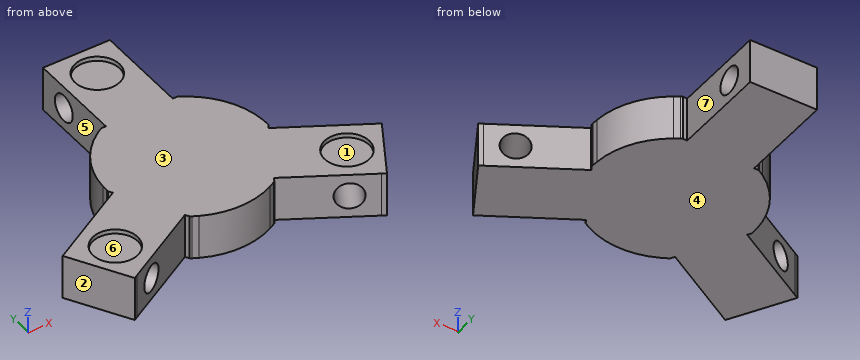
from build123d import *
from build123d.topology import SkipClean

# Parameters (mm, degrees)
EXTRUDE_1_DEPTH      = 5
SKETCH_2_R           = 1.5
CUT_EXTRUDE_1_DEPTH  = 10
SKETCH_3_R           = 1.5
CUT_EXTRUDE_2_DEPTH  = 10
SKETCH_4_R           = 1.5
CUT_EXTRUDE_3_DEPTH  = 10
CUT_EXTRUDE_4_DEPTH  = 3
SKETCH_6_R           = 2.5
CUT_EXTRUDE_5_DEPTH  = 5
CUT_EXTRUDE_START    = -10
CUT_EXTRUDE_6_DEPTH  = 10
SKETCH_9_R           = 2.9
CUT_EXTRUDE_7_DEPTH  = 10
CUT_EXTRUDE_8_DEPTH  = 10
SKETCH_12_R          = 2.5
CUT_EXTRUDE_10_DEPTH = 0.5
SKETCH_13_R          = 5.742346741
EXTRUDE_2_DEPTH      = 5
SKETCH_14_W          = 0.5
SKETCH_14_H          = 10.069998948
CUT_EXTRUDE_11_DEPTH = 5
SKETCH_16_W          = 7.5
SKETCH_16_H          = 0.5
EXTRUDE_3_DEPTH      = 5


with BuildPart() as part:
    # 草图1 → 凸台-拉伸1 (new body)
    with BuildSketch(Plane.XY):
        with BuildLine():
            Line((8.980740698, 0.588469632), (18.088457268, -4.669872981))
            Line((18.088457268, -4.669872981), (13.088457268, -13.330127019))
            Line((13.088457268, -13.330127019), (3.980740698, -8.071784406))
            ThreePointArc((3.980740698, -8.071784406), (0, -9), (-3.980740698, -8.071784406))
            Line((-3.980740698, -8.071784406), (-13.088457268, -13.330127019))
            Line((-13.088457268, -13.330127019), (-18.088457268, -4.669872981))
            Line((-18.088457268, -4.669872981), (-8.980740698, 0.588469632))
            ThreePointArc((-8.980740698, 0.588469632), (-7.794228634, 4.5), (-5, 7.483314774))
            Line((-5, 7.483314774), (-5, 18.003314774))
            Line((-5, 18.003314774), (5, 18.003314774))
            Line((5, 18.003314774), (5, 7.483314774))
            ThreePointArc((5, 7.483314774), (7.794228634, 4.5), (8.980740698, 0.588469632))
        make_face()
    extrude(amount=EXTRUDE_1_DEPTH)

    # 草图2 → 切除-拉伸1 (cut)
    with BuildSketch(Plane(origin=(5, 0, 0), x_dir=(0, 0, -1), z_dir=(1, 0, 0))):
        with Locations(Location((-2.5, 15.003314774, 0), (0, 0, 90))):
            Circle(SKETCH_2_R)
    extrude(amount=-CUT_EXTRUDE_1_DEPTH, mode=Mode.SUBTRACT)

    # 草图3 → 切除-拉伸2 (cut)
    with BuildSketch(Plane(origin=(-2.5, -4.330127019, 0), x_dir=(0.8660254037844364, -0.5000000000000041, 0), z_dir=(-0.500000000000004, -0.8660254037844363, 0))):
        with Locations((15, 2.5)):
            Circle(SKETCH_3_R)
    extrude(amount=-CUT_EXTRUDE_2_DEPTH, mode=Mode.SUBTRACT)

    # 草图4 → 切除-拉伸3 (cut)
    with BuildSketch(Plane(origin=(2.5, -4.330127019, 0), x_dir=(0.8660254037844434, 0.49999999999999184, 0), z_dir=(0.49999999999999184, -0.8660254037844434, 0))):
        with Locations((-15, 2.5)):
            Circle(SKETCH_4_R)
    extrude(amount=-CUT_EXTRUDE_3_DEPTH, mode=Mode.SUBTRACT)

    # 草图5 → 切除-拉伸4 (cut)
    with BuildSketch(Plane.XY.offset(5)):
        Polygon((-4, 0), (-2, -3.464101615), (2, -3.464101615), (4, 0), (2, 3.464101615), (-2, 3.464101615), align=None)
    extrude(amount=-CUT_EXTRUDE_4_DEPTH, mode=Mode.SUBTRACT)

    # 草图6 → 切除-拉伸5 (cut)
    with BuildSketch(Plane.XY.offset(5)):
        Circle(SKETCH_6_R)
    extrude(amount=-CUT_EXTRUDE_5_DEPTH, mode=Mode.SUBTRACT)

    # 草图8 → 切除-拉伸6 (cut)
    with SkipClean():  # the faces are left unmerged after this step: merging them gives an invalid solid
        with BuildSketch(Plane.XY.offset(5).offset(CUT_EXTRUDE_START)):
            with BuildLine():
                Line((-8.999815496, -0.057628503), (-17.813457268, -5.146186953))
                Line((-17.813457268, -5.146186953), (-18.088457268, -4.669872981))
                Line((-18.088457268, -4.669872981), (-8.980740698, 0.588469632))
                ThreePointArc((-8.980740698, 0.588469632), (-8.996080311, 0.265591864), (-8.999815496, -0.057628503))
            make_face()
            with BuildLine():
                Line((-4.549815496, -7.765254597), (-13.363457268, -12.853813047))
                Line((-13.363457268, -12.853813047), (-13.088457268, -13.330127019))
                Line((-13.088457268, -13.330127019), (-3.980740698, -8.071784406))
                ThreePointArc((-3.980740698, -8.071784406), (-4.268030855, -7.923630016), (-4.549815496, -7.765254597))
            make_face()
            with BuildLine():
                Line((-4.45, 7.8228831), (-4.45, 18.003314774))
                Line((-4.45, 18.003314774), (-5, 18.003314774))
                Line((-5, 18.003314774), (-5, 7.483314774))
                ThreePointArc((-5, 7.483314774), (-4.728049456, 7.658038152), (-4.45, 7.8228831))
            make_face()
            with BuildLine():
                Line((4.45, 7.8228831), (4.45, 18.003314774))
                Line((4.45, 18.003314774), (5, 18.003314774))
                Line((5, 18.003314774), (5, 7.483314774))
                ThreePointArc((5, 7.483314774), (4.728049456, 7.658038152), (4.45, 7.8228831))
            make_face()
            with BuildLine():
                Line((4.549815496, -7.765254597), (13.363457268, -12.853813047))
                Line((13.363457268, -12.853813047), (13.088457268, -13.330127019))
                Line((13.088457268, -13.330127019), (3.980740698, -8.071784406))
                ThreePointArc((3.980740698, -8.071784406), (4.268030855, -7.923630016), (4.549815496, -7.765254597))
            make_face()
            with BuildLine():
                Line((8.999815496, -0.057628503), (17.813457268, -5.146186953))
                Line((17.813457268, -5.146186953), (18.088457268, -4.669872981))
                Line((18.088457268, -4.669872981), (8.980740698, 0.588469632))
                ThreePointArc((8.980740698, 0.588469632), (8.996080311, 0.265591864), (8.999815496, -0.057628503))
            make_face()
        extrude(amount=CUT_EXTRUDE_6_DEPTH, mode=Mode.SUBTRACT)

    # 草图9 → 切除-拉伸7 (cut)
    with SkipClean():  # the faces are left unmerged after this step: merging them gives an invalid solid
        with BuildSketch(Plane(origin=(0, 0, 0), x_dir=(-1, 0, 0), z_dir=(0, 0, -1))):
            Circle(SKETCH_9_R)
        extrude(amount=-CUT_EXTRUDE_7_DEPTH, mode=Mode.SUBTRACT)

    # 草图11 → 切除-拉伸8 (cut)
    with BuildSketch(Plane.XY.offset(5).offset(CUT_EXTRUDE_START)):
        with BuildLine():
            Line((17.813457268, -5.146186953), (17.713457268, -5.319392034))
            Line((17.713457268, -5.319392034), (8.995453042, -0.286049947))
            ThreePointArc((8.995453042, -0.286049947), (8.998359102, -0.171853068), (8.999815496, -0.057628503))
            Line((8.999815496, -0.057628503), (17.813457268, -5.146186953))
        make_face()
        with BuildLine():
            Line((-4.45, 18.003314774), (-4.25, 18.003314774))
            Line((-4.25, 18.003314774), (-4.25, 7.933315826))
            ThreePointArc((-4.25, 7.933315826), (-4.350350428, 7.878734109), (-4.45, 7.8228831))
            Line((-4.45, 7.8228831), (-4.45, 18.003314774))
        make_face()
        with BuildLine():
            Line((4.45, 18.003314774), (4.45, 7.8228831))
            ThreePointArc((4.45, 7.8228831), (4.350350428, 7.878734109), (4.25, 7.933315826))
            Line((4.25, 7.933315826), (4.25, 18.003314774))
            Line((4.25, 18.003314774), (4.45, 18.003314774))
        make_face()
        with BuildLine():
            Line((13.363457268, -12.853813047), (4.549815496, -7.765254597))
            ThreePointArc((4.549815496, -7.765254597), (4.648008674, -7.70688104), (4.745453042, -7.647265879))
            Line((4.745453042, -7.647265879), (13.463457268, -12.680607966))
            Line((13.463457268, -12.680607966), (13.363457268, -12.853813047))
        make_face()
        with BuildLine():
            Line((-4.549815496, -7.765254597), (-13.363457268, -12.853813047))
            Line((-13.363457268, -12.853813047), (-13.463457268, -12.680607966))
            Line((-13.463457268, -12.680607966), (-4.745453042, -7.647265879))
            ThreePointArc((-4.745453042, -7.647265879), (-4.648008674, -7.70688104), (-4.549815496, -7.765254597))
        make_face()
        with BuildLine():
            Line((-17.813457268, -5.146186953), (-17.713457268, -5.319392034))
            Line((-17.713457268, -5.319392034), (-8.995453042, -0.286049947))
            ThreePointArc((-8.995453042, -0.286049947), (-8.998359102, -0.171853068), (-8.999815496, -0.057628503))
            Line((-8.999815496, -0.057628503), (-17.813457268, -5.146186953))
        make_face()
    extrude(amount=CUT_EXTRUDE_8_DEPTH, mode=Mode.SUBTRACT)

    # 草图12 → 切除-拉伸10 (cut)
    with BuildSketch(Plane.XY.offset(5)):
        with Locations((0, 15)):
            Circle(SKETCH_12_R)
        with Locations((12.990381057, -7.5)):
            Circle(SKETCH_12_R)
        with Locations((-12.990381057, -7.5)):
            Circle(SKETCH_12_R)
    extrude(amount=-CUT_EXTRUDE_10_DEPTH, mode=Mode.SUBTRACT)

    # 草图13 → 凸台-拉伸2 (add)
    with BuildSketch(Plane.XY.offset(5)):
        Circle(SKETCH_13_R)
    extrude(amount=-EXTRUDE_2_DEPTH)

    # 草图14 → 切除-拉伸11 (cut)
    with BuildSketch(Plane.XY.offset(5)):
        with Locations((-4, 12.9683153)):
            Rectangle(SKETCH_14_W, SKETCH_14_H)
        with Locations((4, 12.9683153)):
            Rectangle(SKETCH_14_W, SKETCH_14_H)
        Polygon((-17.463457268, -5.752404736), (-8.745453042, -0.719062649), (-8.995453042, -0.286049947), (-17.713457268, -5.319392034), align=None)
        Polygon((-4.995453042, -7.214253177), (-13.713457268, -12.247595264), (-13.463457268, -12.680607966), (-4.745453042, -7.647265879), align=None)
        Polygon((13.713457268, -12.247595264), (4.995453042, -7.214253177), (4.745453042, -7.647265879), (13.463457268, -12.680607966), align=None)
        Polygon((8.745453042, -0.719062649), (17.463457268, -5.752404736), (17.713457268, -5.319392034), (8.995453042, -0.286049947), align=None)
    extrude(amount=-CUT_EXTRUDE_11_DEPTH, mode=Mode.SUBTRACT)

    # 草图16 → 凸台-拉伸3 (add)
    with BuildSketch(Plane.XY.offset(5)):
        with Locations((0, 18.253314774)):
            Rectangle(SKETCH_16_W, SKETCH_16_H)
        Polygon((-17.89646997, -6.002404736), (-14.14646997, -12.497595264), (-13.713457268, -12.247595264), (-17.463457268, -5.752404736), align=None)
        Polygon((17.89646997, -6.002404736), (14.14646997, -12.497595264), (13.713457268, -12.247595264), (17.463457268, -5.752404736), align=None)
    extrude(amount=-EXTRUDE_3_DEPTH)


solid = part.part
Could you check a few things on this model? Use its own coordinates, in mm. Face numbers are marked on the shaded views. A direction names the side the tool comes from. Coordinates: 2 decimals unless noted, no trailing zeros. Order: outer loops, then holes, each group sorted by start corner. A loop starts at its lowest first (then second) coordinate and runs counter-clockwise, first axis right, second up. Notation, with made-up numbers: (41.5, -19.5) - (64.5, -19.5) arc R31 cw to (64.5, 18.5) - close; hole circle Ø9 at (69, -16). An arc over 180 degrees is marked (long way). Answer in a Markdown table with one row per item. Add a question column.
(1) If we section it at C-C, the plane z = 0.45: Please give me the cut outline in (x, y).
(2) If we section it at B-B, the plane y = 15: Please give me the cut outline in (x, z).
(3) On a 3-axis mill with a long thin cutter (end or side, diameter ignored), from which of +Z, -Z, +X, -X, +Y, -Y can I reach the whole of each face in a straight line? I mean the marked faces 4, 5, 6 and 7. Say none if no direction works.
(4) If we section it at A-A, the plane x = 0: Please give me the cut outline in (y, z).
(5) If we mould it in two halves opening along Y, with no side actions, what happens to the marked faces 1, 2 and 3? For each: released by +Y, released by -Y, zero draft, split by the parting line, or undercut.
(6) I need wall thicknesses on L1, parallel to X at y = 16.5, z = 3.05; L2, parallel to Y at x = -2, z = 1.35; L3, parallel to X at y = 5.5, z = 0.65. Which ranges of each line are inside material? Lowest first, please.
(7) If we section it at D-D, the plane z = 2.5: State how many separate pieces and enclosed holes the cut face has, then the cut area to 3 significant figures.
(8) Will these pins go through, and if not, where does the flat tip stop? pin 1 (2 mm diameter, centred on y = 3.5, z = 3, fed in from +X); pin 2 (2.5 mm diameter, centred on y = 15, z = 2.5, fed in from +X); pin 3 (2.5 mm diameter, centred on y = 10.5, z = 3.5, fed in from +X); pin 4 (3 mm diameter, centred on y = 8.5, z = 2, fed in from +X).
Results are:
| question | item | result |
|---|---|---|
| 1 | outline | (-17.9, -6) - (-14.15, -12.5) - (-5, -7.21) - (-4.75, -7.65) arc R9 ccw to (-4.55, -7.77) arc R9 ccw to (4.55, -7.77) arc R9 ccw to (4.75, -7.65) - (5, -7.21) - (14.15, -12.5) - (17.9, -6) - (8.75, -0.72) - (9, -0.29) arc R9 ccw to (5, 7.48) arc R9 ccw to (4.45, 7.82) arc R9 ccw to (4.25, 7.93) - (3.75, 7.93) - (3.75, 18.5) - (-3.75, 18.5) - (-3.75, 7.93) - (-4.25, 7.93) arc R9 ccw to (-4.45, 7.82) arc R9 ccw to (-9, -0.06) arc R9 ccw to (-9, -0.29) - (-8.75, -0.72) - close |
| 2 | outline | (-3.75, 0) - (3.75, 0) - (3.75, 1) - (-3.75, 1) - close; (-3.75, 4) - (3.75, 4) - (3.75, 5) - (2.5, 5) - (2.5, 4.5) - (-2.5, 4.5) - (-2.5, 5) - (-3.75, 5) - close |
| 3 | face 4 | -Z, +X, -X, +Y, -Y |
| 3 | face 5 | +Z, -Z, -X, +Y |
| 3 | face 6 | +Z |
| 3 | face 7 | +Z, -Z, +X, +Y |
| 4 | outline | (-9, 0) - (18.5, 0) - (18.5, 5) - (17.5, 5) - (17.5, 4.5) - (12.5, 4.5) - (12.5, 5) - (-9, 5) - close; hole circle Ø3 at (15, 2.5) |
| 5 | face 1 | undercut |
| 5 | face 2 | released by -Y |
| 5 | face 3 | zero draft |
| 6 | L1 | x = -3.75 to 3.75 |
| 6 | L2 | y = -8.77 to 14.04, 15.97 to 18.5 |
| 6 | L3 | x = -7.12 to 7.12 |
| 7 | separate pieces | 4 |
| 7 | enclosed holes | 0 |
| 7 | area | 406 mm2 |
| 8 | pin 1 | stops at x = 8.65 |
| 8 | pin 2 | passes through |
| 8 | pin 3 | stops at x = 3.75 |
| 8 | pin 4 | stops at x = 5.66 |
